Here's how the part is built. I have some questions about the finished solid (model axes, mm). A direction names the side the tool comes from. Round coordinates to 2 decimals unless told otherwise and drop trailing zeros. Loops run counter-clockwise (first coordinate to the right, second up) from the corner with the lowest first, then second, coordinate; pieces in that order, holes last. Notation, with made-up numbers: M -39.75,2 L -13.75,2 A33 cw -13.75,40 Z; hole C 72,-9 d3. An arc over 180 degrees is marked long. Write item = value, one per line. Start each with the question number.
from build123d import *

# Parameters (mm, degrees)
ESQUISSE1_W             = 91
ESQUISSE1_H             = 73.5
ESQUISSE1_R             = 1.5
ESQUISSE1_W_2           = 76
ESQUISSE1_H_2           = 63.5
BOSS_EXTRU_1_DEPTH      = 8
ENL_V_MAT_EXTRU_1_DEPTH = 2
ESQUISSE3_W             = 76
ESQUISSE3_H             = 5
ENL_V_MAT_EXTRU_2_DEPTH = 2.7
BOSS_EXTRU_2_DEPTH      = 73.5
ESQUISSE5_W             = 91
ESQUISSE5_H             = 10
BOSS_EXTRU_3_DEPTH      = 5.3
ESQUISSE6_W             = 5
ESQUISSE6_H             = 10
ESQUISSE6_W_2           = 10
BOSS_EXTRU_4_DEPTH      = 2.7
ESQUISSE7_W             = 4
ESQUISSE7_H             = 4
ENL_V_MAT_EXTRU_3_DEPTH = 92


with BuildPart() as part:
    # Esquisse1 → Boss.-Extru.1 (new body)
    with BuildSketch(Plane(origin=(0, 0, 0), x_dir=(1, 0, 0), z_dir=(0, 1, 0))):
        with Locations((-2.5, 0)):
            Rectangle(ESQUISSE1_W, ESQUISSE1_H)
        with Locations((-42, -25.25)):
            Circle(ESQUISSE1_R, mode=Mode.SUBTRACT)
        Rectangle(ESQUISSE1_W_2, ESQUISSE1_H_2, mode=Mode.SUBTRACT)
    extrude(amount=BOSS_EXTRU_1_DEPTH)

    # Esquisse2 → Enlèv. mat.-Extru.1 (cut)
    with BuildSketch(Plane(origin=(0, 8, 0), x_dir=(1, 0, 0), z_dir=(0, 1, 0))):
        with BuildLine():
            Line((-42, -30.25), (-38, -30.25))
            Line((-38, -30.25), (-38, -20.25))
            Line((-38, -20.25), (-42, -20.25))
            ThreePointArc((-42, -20.25), (-47, -25.25), (-42, -30.25))
        make_face()
    extrude(amount=-ENL_V_MAT_EXTRU_1_DEPTH, mode=Mode.SUBTRACT)

    # Esquisse3 → Enlèv. mat.-Extru.2 (cut)
    with BuildSketch(Plane(origin=(0, 8, 0), x_dir=(1, 0, 0), z_dir=(0, 1, 0))):
        with Locations((0, -34.25)):
            Rectangle(ESQUISSE3_W, ESQUISSE3_H)
        with Locations((0, 34.25)):
            Rectangle(ESQUISSE3_W, ESQUISSE3_H)
    extrude(amount=-ENL_V_MAT_EXTRU_2_DEPTH, mode=Mode.SUBTRACT)

    # Esquisse4 → Boss.-Extru.2 (add)
    with BuildSketch(Plane(origin=(0, 0, -36.75), x_dir=(-1, 0, 0), z_dir=(0, 0, -1))):
        Polygon((-43, 8), (-38, 8), (-38, 24), (-33, 24), (-33, 27), (-38.815944916, 27), (-43, 27), align=None)
    extrude(amount=-BOSS_EXTRU_2_DEPTH)

    # Esquisse5 → Boss.-Extru.3 (add)
    with BuildSketch(Plane.XZ):
        with Locations((-2.5, -41.75)):
            Rectangle(ESQUISSE5_W, ESQUISSE5_H)
        with Locations((-2.5, 41.75)):
            Rectangle(ESQUISSE5_W, ESQUISSE5_H)
    extrude(amount=-BOSS_EXTRU_3_DEPTH)

    # Esquisse6 → Boss.-Extru.4 (add)
    with BuildSketch(Plane(origin=(0, 5.3, 0), x_dir=(1, 0, 0), z_dir=(0, 1, 0))):
        with Locations((40.5, 41.75)):
            Rectangle(ESQUISSE6_W, ESQUISSE6_H)
        with Locations((40.5, -41.75)):
            Rectangle(ESQUISSE6_W, ESQUISSE6_H)
        with Locations((-43, 41.75)):
            Rectangle(ESQUISSE6_W_2, ESQUISSE6_H)
        with Locations((-43, -41.75)):
            Rectangle(ESQUISSE6_W_2, ESQUISSE6_H)
    extrude(amount=BOSS_EXTRU_4_DEPTH)

    # Esquisse7 → Enlèv. mat.-Extru.3 (cut, through all)
    with BuildSketch(Plane.ZY.offset(48)):
        with Locations((-44.75, 3.7)):
            Rectangle(ESQUISSE7_W, ESQUISSE7_H)
        with Locations((44.75, 3.7)):
            Rectangle(ESQUISSE7_W, ESQUISSE7_H)
    extrude(amount=-ENL_V_MAT_EXTRU_3_DEPTH, mode=Mode.SUBTRACT)


solid = part.part
Item 1: I want a section at A-A, the plane x = 20. List the corners of the cut face in (y, z) for me.
Item 2: Please list where these lines run through material, in increasing order: line 1 (X direction, y = 4.5, z = 25.25); line 2 (Z direction, x = -42, y = 4.05); line 3 (Z direction, x = -42, y = 1.25). Write a range as [from, to].
Item 3: Will these pins go through, and if not, where does the flat tip stop? pin 1 Ø2 at (x, y) = (6, 4) entering from +Z; pin 2 Ø1.5 at (x, y) = (32, 24) entering from +Z; pin 3 Ø11 at (x, z) = (-43.5, 1) entering from +Y; pin 4 Ø0.9 at (y, z) = (26, 17) entering from -X.
Item 4: I want a section at B-B, the plane z = 13.5. List the corners of the cut face in (x, y) for me, then the cut area to 3 significant figures.
Item 5: I want a section at C-C, the plane z = 25.25. List the corners of the cut face in (x, y) for me, then the cut area to 3 significant figures.
Item 6: We'd pull the mould along Z, two halves only. Please class faces 4 (the flat face through (-43, 5.7, 45)), 5 (the flat face through (-3, 4, -42.75)), 6 (the flat face through (-1, 3, 31.75)): released by +Z, released by -Z, zero draft, split by the parting line, or undercut.
Item 7: For faces 1 (the flat face through (40, 5.7, -45)), 2 (the flat face through (-3, 4, 42.75)), 3 (the flat face through (-40, 7, 20.25)), which set-ups out of +Z, -Z, +X, -X, +Y, -Y let a thin tool reach every point of the face, with its end or its side?
Worked out:
q1.outline = M 0,-46.75 L 1.7,-46.75 L 1.7,-42.75 L 5.3,-42.75 L 5.3,-31.75 L 0,-31.75 Z; M 0,31.75 L 5.3,31.75 L 5.3,42.75 L 1.7,42.75 L 1.7,46.75 L 0,46.75 Z
q2.line_1 = [-48, -43.5], [-40.5, -38], [38, 43]
q2.line_2 = [-42.75, 23.75], [26.75, 42.75]
q2.line_3 = [-46.75, 23.75], [26.75, 46.75]
q3.pin_1 = 42.75
q3.pin_2 = through
q3.pin_3 = 8
q3.pin_4 = 33
q4.outline = M -48,0 L -38,0 L -38,8 L -48,8 Z; M 33,24 L 38,24 L 38,0 L 43,0 L 43,27 L 33,27 Z
q4.area = 230 mm2
q5.outline = M -48,0 L -43.5,0 L -43.5,6 L -47,6 L -47,8 L -48,8 Z; M -40.5,0 L -38,0 L -38,6 L -40.5,6 Z; M 33,24 L 38,24 L 38,0 L 43,0 L 43,27 L 33,27 Z
q5.area = 194 mm2
q6.face_4 = zero draft
q6.face_5 = released by -Z
q6.face_6 = undercut
q7.face_1 = -Z, +X, -X
q7.face_2 = +Z, +X, -X
q7.face_3 = +Y
